Could you check a few things on this drawing? It's one solid part, dimensions in mm from its lowest x, y, z. A direction names the side the tool comes from. Coordinates: 2 decimals unless noted, no trailing zeros. Write each loop counter-clockwise with the first axis right and the second up, starting at its lowest first coordinate (ties: lowest second). Pieces come first, ordered by that corner, then holes.
Item 1: I want a section at D-D (z = 4). Please give me the cut outline in (x, y), and give its area (3 significant figures).
Item 2: I want a section at B-B (z = 33.5). Please give me the cut outline in (x, y).
Item 3: I'm going to push flat-ended pins straight in: P1, Ø3, axis at x = 33, y = 3.5, coming from the -Z side; P2, Ø0.8, axis at y = 1, z = 4.5, coming from the -X side; P3, Ø1.5, axis at y = 7.5, z = 25.5, coming from the -X side. Where does each tip first touch, or does it pass through?
Item 4: Please list where these lines run through material, in increasing order: line 1 (Y direction, x = 28, z = 15); line 2 (Z direction, x = 38, y = 2.25); line 3 (X direction, y = 2.5, z = 18.5).
Item 5: I want a section at C-C (y = 7.5). Please give me the cut outline in (x, z).
Item 6: For the marked faces 1 and 2, which set-ups out of +Z, -Z, +X, -X, +Y, -Y let a thin tool reach every point of the face, with its end or its side?
Item 7: I want a section at A-A (x = 21.5). Please give me the cut outline in (y, z), and give its area (3 significant figures).
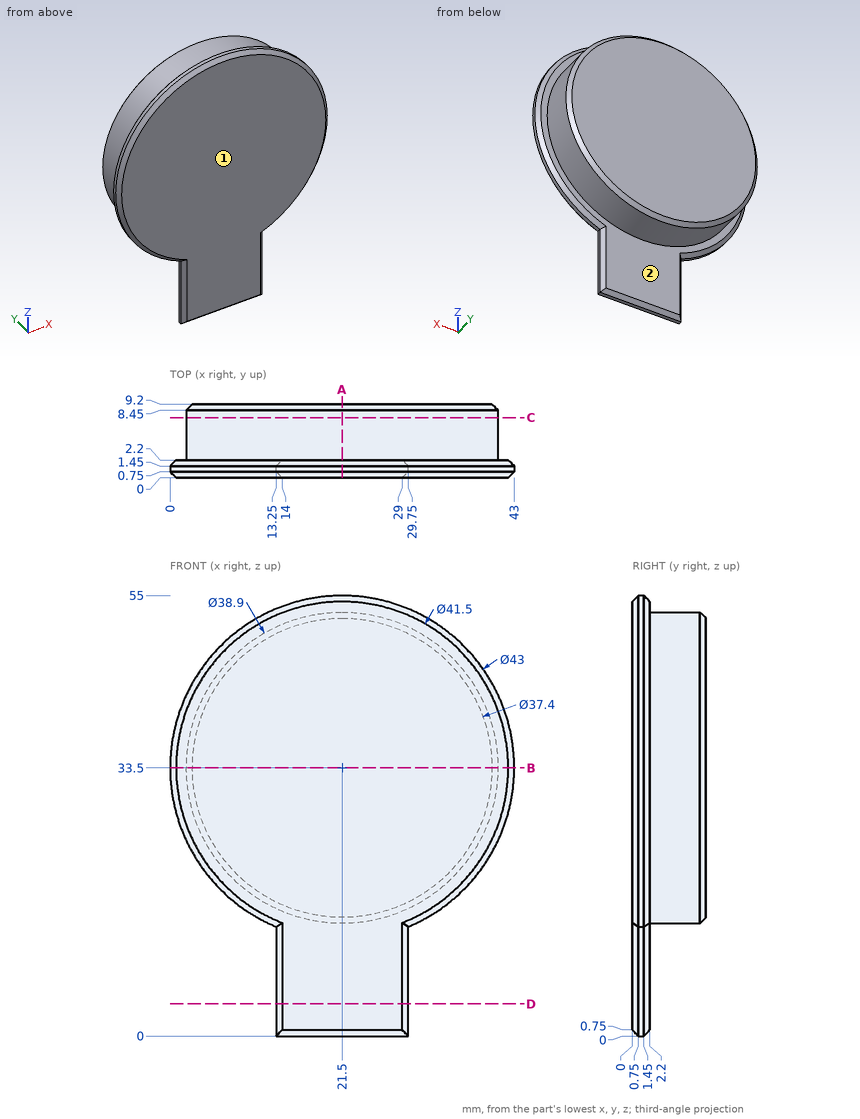
Answer:
1. outline: (13.25, 0.75) - (14, 0) - (29, 0) - (29.75, 0.75) - (29.75, 1.45) - (29, 2.2) - (14, 2.2) - (13.25, 1.45) - close
1. area: 35.2 mm2
2. outline: (0, 0.75) - (0.75, 0) - (42.25, 0) - (43, 0.75) - (43, 1.45) - (42.25, 2.2) - (40.95, 2.2) - (40.95, 8.45) - (40.2, 9.2) - (2.8, 9.2) - (2.05, 8.45) - (2.05, 2.2) - (0.75, 2.2) - (0, 1.45) - close
3. P1: stops at z = 15.75
3. P2: stops at x = 13.25
3. P3: stops at x = 3.45
4. line 1: y = 0 to 2.2
4. line 2: z = 23.2 to 43.8
4. line 3: x = 9.12 to 33.88
5. outline: circle Ø38.9 at (21.5, 33.5)
6. face 1: +Z, -Z, +X, -X, -Y
6. face 2: +Y
7. outline: (0, 0.75) - (0.75, 0) - (1.45, 0) - (2.2, 0.75) - (2.2, 14.05) - (8.45, 14.05) - (9.2, 14.8) - (9.2, 52.2) - (8.45, 52.95) - (2.2, 52.95) - (2.2, 54.25) - (1.45, 55) - (0.75, 55) - (0, 54.25) - close
7. area: 392 mm2
